Read the model definition and answer for the solid it produces. Units are mm, in the model's axes. Face numbers are marked on the shaded views. A direction names the side the tool comes from. Give positions to 0.01 mm unless a question says otherwise; leave off trailing zeros. Order: outer loops, then holes, each group sorted by start corner. A loop starts at its lowest first (then second) coordinate and runs counter-clockwise, first axis right, second up. Notation, with made-up numbers: (84.25, 10) -> (133.25, 10) arc R22 cw to (133.25, 26) -> close; hole circle Ø9 at (51, 70.5). An arc over 180 degrees is marked (long way). Use one line per item in the form item = value.
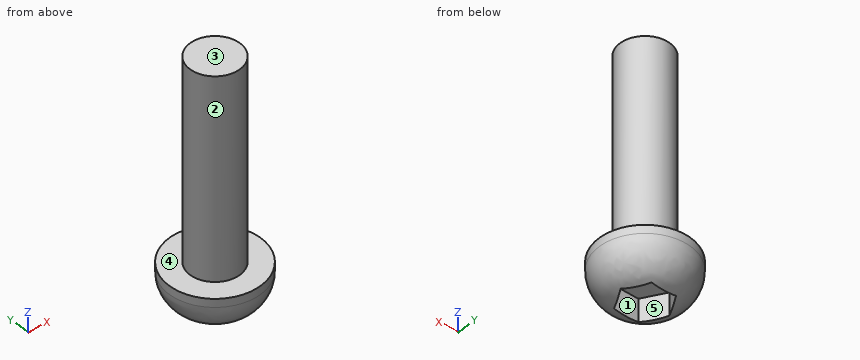
Autodesk Inventor part; units mm, degrees
ref_plane "YZ Plane" through (0, 0, 0) normal (1, 0, 0) x (0, 1, 0)
ref_plane "XZ Plane" through (0, 0, 0) normal (0, 1, 0) x (-1, 0, 0)
ref_plane "XY Plane" through (0, 0, 0) normal (0, 0, 1) x (1, 0, 0)
sketch "Boceto1" plane through (0, 0, 0) normal (0, 0, 1) x (1, 0, 0)
  circle A0 centre (0, 0) radius 1.5
  circle A1 centre (0, 0) radius 2.75
  dimension "d0" = 3
  dimension "d1" = 5.5
extrude "Extrusión1" add sketch "Boceto1" along normal blind 12 contours A0
extrude "Extrusión2" add sketch "Boceto1" against normal blind 2.5 contours A0 | A1
sketch "Boceto2" plane through (0, 0, -2.5) normal (0, 0, -1) x (-1, 0, 0)
  line L0 (1.5, 0) -> (0.75, -1.299)
  line L1 (0.75, -1.299) -> (-0.75, -1.299)
  line L2 (-0.75, -1.299) -> (-1.5, 0)
  line L3 (-1.5, 0) -> (-0.75, 1.299)
  line L4 (-0.75, 1.299) -> (0.75, 1.299)
  line L5 (0.75, 1.299) -> (1.5, 0)
  point P0 (0, 0)
  point P1 (0, 0)
  dimension "d6" = 3
fillet "Empalme1" radius 2 1 edges at (-2.75, 0, -2.5)
extrude "Extrusión4" cut sketch "Boceto2" against normal blind 1.5
thread "Rosca1"
properties part number "tonrilloM3x12mm" material "Aluminio 6061-AHC"
Item 1: The part is cut by section A-A on z = 3.5. Give the vertices of the cut face in (x, y), and give its area (3 significant figures).
Checks:
outline = circle Ø3 at (0, 0)
area = 7.07 mm²
Item 2: Given pin 1 Ø1.6 at (x, z) = (0.5, -1.5) entering from -Y; pin 2 Ø3 at (x, z) = (2, 0.5) entering from +Y; pin 3 Ø0.7 at (x, z) = (0, -2) entering from +Y, each flat-ended and moving along its own axis, determine where each tip first touches the part or whether it passes through.
Checks:
pin_1 = -2.73
pin_2 = 2.69
pin_3 = 2.39
Item 3: Straight lines are drawn through the part: L1, parallel to X at y = 1, z = -1.5; L2, parallel to Y at x = -0.75, z = 0.5; L3, parallel to Z at x = 1, y = -0.15. For each, find the intervals that lie inside material, in ascending order. Write a range as from..to.
Checks:
L1 = -2.27..-0.92, 0.92..2.27
L2 = -1.3..1.3
L3 = -1..12
Item 4: Determine the mould class of the marked faces 1, 2 and 3 for opening direction X: +X half, -X half, draft (parallel to the pull), parting line (faces both ways), or undercut.
Checks:
face_1 = undercut
face_2 = parting line
face_3 = draft
Item 5: Which of the six approach directions +Z, -Z, +X, -X, +Y, -Y give full straight-line access (tool end or side, diameter ignored) to the marked faces 4 and 5?
Checks:
face_4 = +Z
face_5 = -Z
